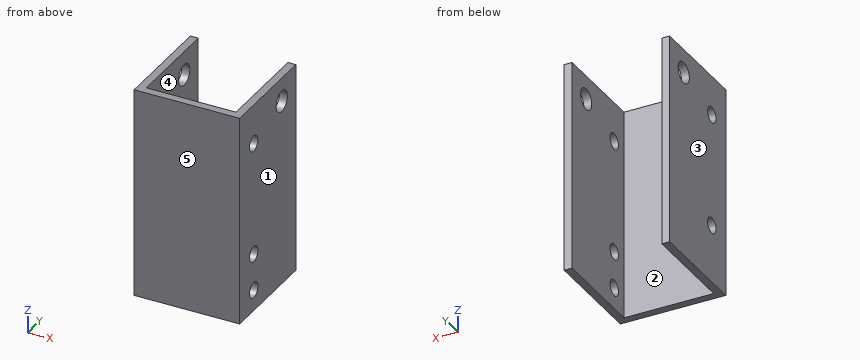
from build123d import *

# Parameters (mm, degrees)
EXTRUSION1_DEPTH = 40
ESQUISSE2_R      = 1.5
ESQUISSE2_R_2    = 2
EXTRUSION2_DEPTH = 49.396797415
ESQUISSE3_R      = 1.5
EXTRUSION3_DEPTH = 6


with BuildPart() as part:
    # Esquisse1 → Extrusion1 (new body)
    with BuildSketch(Plane.XY):
        Polygon((-8.904835854, 18.5), (-8.904835854, -1.5), (11.095164146, -1.5), (11.095164146, 18.5), (9.595164146, 18.5), (9.595164146, 0), (-7.404835854, 0), (-7.404835854, 18.5), align=None)
    extrude(amount=EXTRUSION1_DEPTH)

    # Esquisse2 → Extrusion2 (cut, through all)
    with BuildSketch(Plane(origin=(11.095164146, 0, 0), x_dir=(0, 0, -1), z_dir=(1, 0, 0))):
        with Locations((-32.5, 3.5)):
            Circle(ESQUISSE2_R)
        with Locations((-11, 3.5)):
            Circle(ESQUISSE2_R)
        with Locations((-35.5, 13.5)):
            Circle(ESQUISSE2_R_2)
    extrude(amount=-EXTRUSION2_DEPTH, mode=Mode.SUBTRACT)

    # Esquisse3 → Extrusion3 (cut)
    with BuildSketch(Plane(origin=(11.095164146, 0, 0), x_dir=(0, 0, -1), z_dir=(1, 0, 0))):
        with Locations((-4, 3.5)):
            Circle(ESQUISSE3_R)
    extrude(amount=-EXTRUSION3_DEPTH, mode=Mode.SUBTRACT)


solid = part.part
Geometry: final body of the model. Coordinates: model frame, mm. Face numbers are marked on the shaded views. A direction names the side the tool comes from. Give positions to 0.01 mm unless a question says otherwise; leave off trailing zeros. Write each loop counter-clockwise with the first axis right and the second up, starting at its lowest first coordinate (ties: lowest second). Pieces come first, ordered by that corner, then holes.
(1) Cut plane C-C, the plane y = 8.25. Return loops of the section in (x, z), then the cut area to 3 significant figures.
(2) Cut plane D-D, the plane z = 4. Return loops of the section in (x, y), then the cut area to 3 significant figures.
(3) Cut plane A-A, the plane y = 13.5. Return loops of the section in (x, z).
(4) Cut plane B-B, the plane z = 32.5. Return loops of the section in (x, y).
(5) First-contact query: P1, Ø1.8, axis at y = 3.5, z = 11, coming from the +X side; P2, Ø8.5, axis at x = 5, z = 25, coming from the +Y side. Flat tips, straight axial feed; report the tip coordinate or a pass-through.
(6) Mould query, pull axis X, two halves, no side actions, for the marked faces 3, 4 and 5. Classes: released by +X, released by -X, zero draft, split by the parting line, or undercut.
(7) Ray query, line 1 (Y direction, x = 10.25, z = 11); line 2 (X direction, y = 16.5, z = 18); line 3 (Y direction, x = -4.5, z = 17). Return the intervals inside material, ascending.
(8) Access query for the marked faces 1 and 2. Directions: +Z, -Z, +X, -X, +Y, -Y. A direction counts if a zero-diameter tool reaches every point of the face in a straight line with its end or side. Return the directions, or none.
Values follow:
1. outline: (-8.9, 0) - (-7.4, 0) - (-7.4, 40) - (-8.9, 40) - close; (9.6, 0) - (11.1, 0) - (11.1, 40) - (9.6, 40) - close
1. area: 120 mm2
2. outline: (-8.9, -1.5) - (11.1, -1.5) - (11.1, 2) - (9.6, 2) - (9.6, 0) - (-7.4, 0) - (-7.4, 18.5) - (-8.9, 18.5) - close; (9.6, 5) - (11.1, 5) - (11.1, 18.5) - (9.6, 18.5) - close
2. area: 81.0 mm2
3. outline: (-8.9, 0) - (-7.4, 0) - (-7.4, 33.5) - (-8.9, 33.5) - close; (-8.9, 37.5) - (-7.4, 37.5) - (-7.4, 40) - (-8.9, 40) - close; (9.6, 0) - (11.1, 0) - (11.1, 33.5) - (9.6, 33.5) - close; (9.6, 37.5) - (11.1, 37.5) - (11.1, 40) - (9.6, 40) - close
4. outline: (-8.9, -1.5) - (11.1, -1.5) - (11.1, 2) - (9.6, 2) - (9.6, 0) - (-7.4, 0) - (-7.4, 2) - (-8.9, 2) - close; (-8.9, 5) - (-7.4, 5) - (-7.4, 18.5) - (-8.9, 18.5) - close; (9.6, 5) - (11.1, 5) - (11.1, 18.5) - (9.6, 18.5) - close
5. P1: passes through
5. P2: stops at y = 0
6. face 3: released by -X
6. face 4: undercut
6. face 5: zero draft
7. line 1: y = -1.5 to 2, 5 to 18.5
7. line 2: x = -8.9 to -7.4, 9.6 to 11.1
7. line 3: y = -1.5 to 0
8. face 1: +Z, -Z, +X, +Y, -Y
8. face 2: +Z, -Z, +Y
